Autodesk Inventor part; units mm, degrees
ref_plane "YZ Plane" through (0, 0, 0) normal (1, 0, 0) x (0, 1, 0)
ref_plane "XZ Plane" through (0, 0, 0) normal (0, 1, 0) x (-1, 0, 0)
ref_plane "XY Plane" through (0, 0, 0) normal (0, 0, 1) x (1, 0, 0)
sketch "草圖1" plane through (0, 0, 0) normal (1, 0, 0) x (0, 1, 0)
  line L0 (-112.5, 112.5) -> (112.5, 112.5)
  line L1 (112.5, 112.5) -> (112.5, -112.5)
  line L2 (112.5, -112.5) -> (-112.5, -112.5)
  line L3 (-112.5, -112.5) -> (-112.5, 112.5)
  line L4 (-112.5, 112.5) -> (112.5, -112.5) construction
  line L5 (112.5, 112.5) -> (-112.5, -112.5) construction
  point P0 (0, 0)
  dimension "d0" = 225
  dimension "d1" = 225
extrude "擠出1" add sketch "草圖1" along normal blind 20
fillet "圓角1" radius 30 4 edges at (10, 112.5, 112.5) (10, -112.5, 112.5) (10, 112.5, -112.5) (10, -112.5, -112.5)
chamfer "倒角1" distance 10 angle 45 8 edges at (20, 0, 112.5) (20, -103.7132, 103.7132) (20, -112.5, 0) (20, -103.7132, -103.7132) (20, 0, -112.5) (20, 103.7132, -103.7132) (20, 112.5, 0) (20, 103.7132, 103.7132)
sketch "草圖2" plane through (20, 0, 0) normal (1, 0, 0) x (0, 0, -1)
  line L0 (-62.5, -62.5) -> (62.5, -62.5)
  line L1 (62.5, -62.5) -> (62.5, 62.5)
  line L2 (62.5, 62.5) -> (-62.5, 62.5)
  line L3 (-62.5, 62.5) -> (-62.5, -62.5)
  line L4 (-62.5, -62.5) -> (62.5, 62.5) construction
  line L5 (62.5, -62.5) -> (-62.5, 62.5) construction
  point P0 (0, 0)
  dimension "d8" = 125
  dimension "d9" = 125
hole "孔1" at (20, 62.5, 62.5) at (20, 62.5, -62.5) at (20, -62.5, 62.5) at (20, -62.5, -62.5) direction (-1, 0, 0) diameter 12 depth 10 tip angle 118
sketch "草圖3" plane through (0, 0, 0) normal (-1, 0, 0) x (0, 0, 1)
  arc A0 (-112.5, -82.5) -> (-82.5, -112.5) centre (-82.5, -82.5) ccw
  line L0 (-82.5, -112.5) -> (82.5, -112.5)
  arc A1 (82.5, -112.5) -> (112.5, -82.5) centre (82.5, -82.5) ccw
  line L1 (112.5, -82.5) -> (112.5, 82.5)
  arc A2 (112.5, 82.5) -> (82.5, 112.5) centre (82.5, 82.5) ccw
  line L2 (82.5, 112.5) -> (-82.5, 112.5)
  arc A3 (-82.5, 112.5) -> (-112.5, 82.5) centre (-82.5, 82.5) ccw
  line L3 (-112.5, 82.5) -> (-112.5, -82.5)
  line L4 (87.5, 87.5) -> (-87.5, 87.5)
  line L5 (-87.5, 87.5) -> (-87.5, -87.5)
  line L6 (-87.5, -87.5) -> (87.5, -87.5)
  line L7 (87.5, -87.5) -> (87.5, 87.5)
  line L8 (87.5, 87.5) -> (-87.5, -87.5) construction
  line L9 (-87.5, 87.5) -> (87.5, -87.5) construction
  point P0 (0, 0)
  dimension "d17" = 175
  dimension "d18" = 175
hole "孔2" at (0, -87.5, 87.5) at (0, -87.5, -87.5) at (0, 87.5, -87.5) at (0, 87.5, 87.5) direction (1, 0, 0) diameter 12 depth 10 tip angle 118
properties part number "exercise3-1-3"
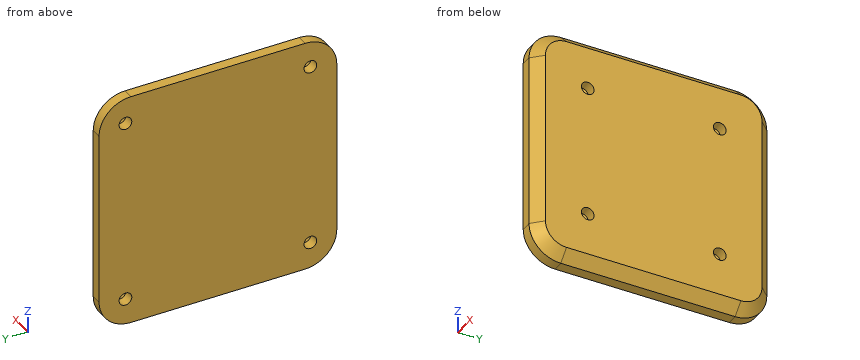
Read the model definition and answer for the solid it produces. Units are mm, in the model's axes. Coordinates: 2 decimals unless noted, no trailing zeros. Write each loop counter-clockwise with the first axis right and the second up, starting at its lowest first coordinate (ties: lowest second). Pieces come first, ordered by that corner, then holes. Notation, with made-up numbers: M 87,35.25 L 119,35.25 A18 ccw 119,42.25 Z; hole C -19.75,33 d6. An arc over 180 degrees is marked long. Use a Markdown table: item, result.
Q1. Each of these flat-tipped pins is pushed along its axis until it touches: pin 1 Ø2 at (x, z) = (14, -18.5) entering from +Y; pin 2 Ø9.5 at (y, z) = (62.5, -62.5) entering from -X; pin 3 Ø7 at (y, z) = (62.5, 62.5) entering from +X. Where does it stop, or does it pass through?
Answer block:
| item | result |
|---|---|
| pin 1 | stops at y = 109.5 |
| pin 2 | stops at x = 0 |
| pin 3 | stops at x = 8.5 |
Q2. Straight lines are drawn through the part: L1, parallel to Z at x = 13.75, y = 62.5; L2, parallel to Y at x = 14, z = -62.5; L3, parallel to Y at x = 6.5, z = 87.5. For each, find the intervals that lie inside material, in ascending order. Write a range as [from, to].
Answer block:
| item | result |
|---|---|
| L1 | z = [-108.75, -68.5], [-56.5, 56.5], [68.5, 108.75] |
| L2 | y = [-108.5, -68.5], [-56.5, 56.5], [68.5, 108.5] |
| L3 | y = [-112.08, -93.5], [-81.5, 81.5], [93.5, 112.08] |
Q3. The part is cut by section A-A, the plane x = 3.25. Write down the section's boundary in (y, z), then the cut area to 3 significant figures.
Answer block:
| item | result |
|---|---|
| outline | M -112.5,-82.5 A30 ccw -82.5,-112.5 L 82.5,-112.5 A30 ccw 112.5,-82.5 L 112.5,82.5 A30 ccw 82.5,112.5 L -82.5,112.5 A30 ccw -112.5,82.5 Z; hole C -87.5,-87.5 d12; hole C -87.5,87.5 d12; hole C 87.5,-87.5 d12; hole C 87.5,87.5 d12 |
| area | 49,400 mm2 |
Q4. The part is cut by section B-B, the plane z = -47. Write down the section's boundary in (x, y), then the cut area to 3 significant figures.
Answer block:
| item | result |
|---|---|
| outline | M 0,-112.5 L 10,-112.5 L 20,-102.5 L 20,102.5 L 10,112.5 L 0,112.5 Z |
| area | 4,400 mm2 |
